```python
from build123d import *

# Parameters (mm, degrees)
SKETCH1_R                       = 10
SKETCH1_R_2                     = 9
EXTRUDE_THIN1_DEPTH             = 2114
F_10_CLEARANCE_HOLE1_AT_2_COUNT = 2
F_10_CLEARANCE_HOLE1_AT_2_PITCH = 54
LPATTERN1_COUNT                 = 4
LPATTERN1_PITCH                 = 616


with BuildPart() as part:
    # Sketch1 → Extrude-Thin1 (new body)
    with BuildSketch(Plane.XY):
        Circle(SKETCH1_R)
        Circle(SKETCH1_R_2, mode=Mode.SUBTRACT)
    extrude(amount=EXTRUDE_THIN1_DEPTH)

    # Sketch4 → #10 Clearance Hole1 (revolve, cut)
    with BuildSketch(Plane(origin=(0, 10, 181.1), x_dir=(0, 0, 1), z_dir=(1, 0, 0))):
        Polygon((0, 0), (0, 11.533816902), (2.5527, 10), (2.5527, 0), align=None)
    f_10_clearance_hole1 = revolve(axis=Axis((0, 16.35, 181.1), (0, -1, 0)), mode=Mode.SUBTRACT)

    # #10 Clearance Hole1 at 2: #10 Clearance Hole1 ×2
    with Locations(*[(0, 0, i * F_10_CLEARANCE_HOLE1_AT_2_PITCH) for i in range(1, F_10_CLEARANCE_HOLE1_AT_2_COUNT)]):
        add(f_10_clearance_hole1, mode=Mode.SUBTRACT)

    # LPattern1: #10 Clearance Hole1 ×4
    with Locations(*[(0, 0, i * LPATTERN1_PITCH) for i in range(1, LPATTERN1_COUNT)]):
        add(f_10_clearance_hole1, mode=Mode.SUBTRACT)

    # LPattern1 copy 1 sketch → LPattern1 copy 1 (revolve, cut)
    with BuildSketch(Plane(origin=(0, 10, 851.1), x_dir=(0, 0, 1), z_dir=(1, 0, 0))):
        Polygon((0, 0), (0, 11.533816902), (2.5527, 10), (2.5527, 0), align=None)
    revolve(axis=Axis((0, 16.35, 851.1), (0, -1, 0)), mode=Mode.SUBTRACT)

    # LPattern1 copy 2 sketch → LPattern1 copy 2 (revolve, cut)
    with BuildSketch(Plane(origin=(0, 10, 1467.1), x_dir=(0, 0, 1), z_dir=(1, 0, 0))):
        Polygon((0, 0), (0, 11.533816902), (2.5527, 10), (2.5527, 0), align=None)
    revolve(axis=Axis((0, 16.35, 1467.1), (0, -1, 0)), mode=Mode.SUBTRACT)

    # LPattern1 copy 3 sketch → LPattern1 copy 3 (revolve, cut)
    with BuildSketch(Plane(origin=(0, 10, 2083.1), x_dir=(0, 0, 1), z_dir=(1, 0, 0))):
        Polygon((0, 0), (0, 11.533816902), (2.5527, 10), (2.5527, 0), align=None)
    revolve(axis=Axis((0, 16.35, 2083.1), (0, -1, 0)), mode=Mode.SUBTRACT)


solid = part.part
```
Part model, mm, in its own coordinate system. Round coordinates to 2 decimals unless told otherwise and drop trailing zeros. Loops run counter-clockwise (first coordinate to the right, second up) from the corner with the lowest first, then second, coordinate; pieces in that order, holes last. Notation, with made-up numbers: (-3, 67.25) -> (26, 67.25) arc R15 cw to (26, 71.25) -> close; hole circle Ø8 at (15.5, 54.25). An arc over 180 degrees is marked (long way). Use CSV: the item, a comma, the result in double quotes. Start each with the question number.
1) Cut at B-B, the plane z = 1976.5. Write the cut outline in (x, y).
2) Cut at A-A, the plane y = 0. Write the cut outline in (x, z).
3) Drop flat-ended pins along their axis: P1, Ø2, axis at x = 6.5, y = 5, coming from the -Z side; P2, Ø2, axis at x = 6, z = 461.5, coming from the +Y side; P3, Ø6, axis at y = 5, z = 1566.5, coming from the -X side. Give the stop position or say it passes through.
4) Wall check: L1, parallel to Y at x = -1, z = 386.5; L2, parallel to X at y = -0.5, z = 1554; L3, parallel to X at y = 2, z = 1022.5. Give the ranges that are in metal, low to high. Write a range as [from, to].
Determined:
1,outline,"circle Ø20 at (0, 0); hole circle Ø18 at (0, 0)"
2,outline,"(-10, 0) -> (-9, 0) -> (-9, 2114) -> (-10, 2114) -> close; (9, 0) -> (10, 0) -> (10, 2114) -> (9, 2114) -> close"
3,P1,"stops at z = 0"
3,P2,"stops at y = 8.66"
3,P3,"stops at x = -9.8"
4,L1,"y = [-9.95, -8.94], [8.94, 9.95]"
4,L2,"x = [-9.99, -8.99], [8.99, 9.99]"
4,L3,"x = [-9.8, -8.77], [8.77, 9.8]"
